```python
from build123d import *

# Parameters (mm, degrees)
BOSS_EXTRUDE1_DEPTH   = 10
SKETCH1_R             = 3.5
BOSS_EXTRUDE1_2_DEPTH = 10
BOSS_EXTRUDE2_DEPTH   = 5
SKETCH1_6_W           = 10
SKETCH1_6_H           = 20
SKETCH1_6_W_2         = 20
SKETCH1_6_H_2         = 2
BOSS_EXTRUDE3_DEPTH   = 1
SKETCH1_7_R           = 8.5
SKETCH1_7_R_2         = 3.5
CUT_EXTRUDE1_DEPTH    = 8
SKETCH2_R             = 10.261268268
SKETCH2_R_2           = 10.194878558
CUT_EXTRUDE4_DEPTH    = 8


with BuildPart() as part:
    # Sketch1 → Boss-Extrude1 (new body)
    with BuildSketch(Plane(origin=(0, 0, 0), x_dir=(1, 0, 0), z_dir=(0, 1, 0))):
        Polygon((0, -102), (0, 0), (102, 0), (102, -102), (61, -102), (61, -104), (104, -104), (104, 2), (-2, 2), (-2, -104), (41, -104), (41, -102), align=None)
    extrude(amount=BOSS_EXTRUDE1_DEPTH)



with BuildPart() as body_2:
    # Sketch1 → Boss-Extrude1 2 (new body)
    with BuildSketch(Plane(origin=(0, 0, 0), x_dir=(1, 0, 0), z_dir=(0, 1, 0))):
        Polygon((2, -100), (41, -100), (41, -80), (61, -80), (61, -100), (100, -100), (100, -2), (2, -2), align=None)
        with Locations((18.5, -12)):
            Circle(SKETCH1_R, mode=Mode.SUBTRACT)
        with Locations((83.5, -12)):
            Circle(SKETCH1_R, mode=Mode.SUBTRACT)
        with Locations((18.5, -52)):
            Circle(SKETCH1_R, mode=Mode.SUBTRACT)
        with Locations((83.5, -52)):
            Circle(SKETCH1_R, mode=Mode.SUBTRACT)
    extrude(amount=BOSS_EXTRUDE1_2_DEPTH)


with BuildPart() as part_1:
    add(part.part)

    add(body_2.part)  # Boss-Extrude2 merges body 2
    # Sketch1_5 → Boss-Extrude2 (add)
    with BuildSketch(Plane(origin=(0, 0, 0), x_dir=(1, 0, 0), z_dir=(0, 1, 0))):
        Polygon((102, 0), (0, 0), (0, -102), (41, -102), (41, -100), (2, -100), (2, -2), (100, -2), (100, -100), (61, -100), (61, -102), (102, -102), align=None)
    extrude(amount=BOSS_EXTRUDE2_DEPTH)

    # Sketch1_6 → Boss-Extrude3 (add)
    with BuildSketch(Plane(origin=(0, 0, 0), x_dir=(1, 0, 0), z_dir=(0, 1, 0))):
        with Locations((46, -90)):
            Rectangle(SKETCH1_6_W, SKETCH1_6_H)
        with Locations((56, -90)):
            Rectangle(SKETCH1_6_W, SKETCH1_6_H)
        Polygon((41, -100), (41, -102), (61, -102), (61, -100), (51, -100), align=None)
        with Locations((51, -103)):
            Rectangle(SKETCH1_6_W_2, SKETCH1_6_H_2)
    extrude(amount=BOSS_EXTRUDE3_DEPTH)

    # Sketch1_7 → Cut-Extrude1 (cut)
    with BuildSketch(Plane(origin=(0, 0, 0), x_dir=(1, 0, 0), z_dir=(0, 1, 0))):
        with Locations((18.5, -52)):
            Circle(SKETCH1_7_R)
        with Locations((18.5, -52)):
            Circle(SKETCH1_7_R_2, mode=Mode.SUBTRACT)
        with Locations((83.5, -52)):
            Circle(SKETCH1_7_R)
        with Locations((83.5, -52)):
            Circle(SKETCH1_7_R_2, mode=Mode.SUBTRACT)
        with Locations((83.5, -12)):
            Circle(SKETCH1_7_R)
        with Locations((83.5, -12)):
            Circle(SKETCH1_7_R_2, mode=Mode.SUBTRACT)
        with Locations((18.5, -12)):
            Circle(SKETCH1_7_R)
        with Locations((18.5, -12)):
            Circle(SKETCH1_7_R_2, mode=Mode.SUBTRACT)
    extrude(amount=CUT_EXTRUDE1_DEPTH, mode=Mode.SUBTRACT)

    # Sketch2 → Cut-Extrude4 (cut)
    with BuildSketch(Plane.XZ):
        with BuildLine():
            Line((98, 4.574503774), (98, 98))
            Line((98, 98), (63, 98))
            Line((63, 98), (63, 76))
            Line((63, 76), (51, 76))
            Line((51, 76), (39, 76))
            Line((39, 76), (39, 98))
            Line((39, 98), (4, 98))
            Line((4, 98), (4, 4.574503774))
            Line((4, 4.574503774), (10.545814352, 4.574503774))
            ThreePointArc((10.545814352, 4.574503774), (14.509161453, 22.123253983), (29.381500977, 12))
            ThreePointArc((29.381500977, 12), (28.623253983, 8.009161453), (26.454185648, 4.574503774))
            Line((26.454185648, 4.574503774), (76.37304098, 4.574503774))
            ThreePointArc((76.37304098, 4.574503774), (79.46399305, 21.467955797), (93.792304848, 12))
            ThreePointArc((93.792304848, 12), (92.967955797, 7.96399305), (90.62695902, 4.574503774))
            Line((90.62695902, 4.574503774), (98, 4.574503774))
        make_face()
        with Locations((18.5, 52)):
            Circle(SKETCH2_R, mode=Mode.SUBTRACT)
        with Locations((83.5, 52)):
            Circle(SKETCH2_R_2, mode=Mode.SUBTRACT)
    extrude(amount=-CUT_EXTRUDE4_DEPTH, mode=Mode.SUBTRACT)


solid = part_1.part
```
The listing builds one solid part. Answer for the finished solid, in the listing's coordinates (mm). A direction names the side the tool comes from. Round coordinates to 2 decimals unless told otherwise and drop trailing zeros. Loops run counter-clockwise (first coordinate to the right, second up) from the corner with the lowest first, then second, coordinate; pieces in that order, holes last.
Q1. Section A-A, the plane y = 3 is taken. Determine the outline of the cut face in (x, z), then the cut area to 3 significant figures.
Q2. Which of the six approach directions +Z, -Z, +X, -X, +Y, -Y give full straight-line access (tool end or side, diameter ignored) to faces 3 (the face through (27.2, 10, -0.3)), 4 (the face through (15, 0, 44)), 5 (the face through (51, 1, 92)), 6 (the face through (51, 4, 76)), 7 (the face through (102, 7, 50))?
Q3. Section C-C, the plane z = 52 is taken. Count the separate pieces of the cut face and the enclosed holes in it, then the cut area to 3 significant figures.
Q4. Given pin 1 Ø22 at (x, z) = (18.5, 52) entering from +Y; pin 2 Ø2.5 at (x, y) = (54.5, 7) entering from +Z; pin 3 Ø8 at (x, z) = (85, 75.5) entering from -Y, each flat-ended and moving along its own axis, determine where each tip first touches the part or whether it passes through.
Q5. Find the intervals of material crossed by line 1 (Z direction, x = 33.5, y = 9); line 2 (X direction, y = 9.5, z = 83), in increasing order.
Q6. For a pull along Z with two mould halves and no side action, classify faces 1 (the face through (55, 0, 78)), 2 (the face through (75, 4, 12)) as released by +Z, released by -Z, zero draft, split by the parting line, or undercut.
Q7. Section B-B, the plane x = 68 is taken. Determine the outline of the cut face in (y, z).
Completed:
1. outline: (-2, -2) - (104, -2) - (104, 104) - (61, 104) - (61, 80) - (41, 80) - (41, 104) - (-2, 104) - close; circle Ø20.52 at (18.5, 52); circle Ø20.39 at (83.5, 52); hole (4, 4.57) - (10.55, 4.57) arc R10.88 cw (long way) to (26.45, 4.57) - (76.37, 4.57) arc R10.29 cw (long way) to (90.63, 4.57) - (98, 4.57) - (98, 98) - (63, 98) - (63, 76) - (39, 76) - (39, 98) - (4, 98) - close; hole circle Ø17 at (18.5, 12); hole circle Ø17 at (18.5, 52); hole circle Ø17 at (83.5, 12); hole circle Ø17 at (83.5, 52)
1. area: 2,890 mm2
2. face 3: +Z, -Z, +X, -X, +Y
2. face 4: +Z, -Z, +X, -X, -Y
2. face 5: +Z, +Y
2. face 6: -Y
2. face 7: +Y
3. separate pieces: 3
3. enclosed holes: 0
3. area: 315 mm2
4. pin 1: stops at y = 10
4. pin 2: stops at z = 80
4. pin 3: stops at y = 8
5. line 1: z = -2 to 0, 2 to 100, 102 to 104
5. line 2: x = -2 to 0, 2 to 41, 61 to 100, 102 to 104
6. face 1: zero draft
6. face 2: undercut
7. outline: (0, -2) - (10, -2) - (10, 0) - (5, 0) - (5, 2) - (10, 2) - (10, 100) - (5, 100) - (5, 102) - (10, 102) - (10, 104) - (0, 104) - (0, 98) - (8, 98) - (8, 4.57) - (0, 4.57) - close
